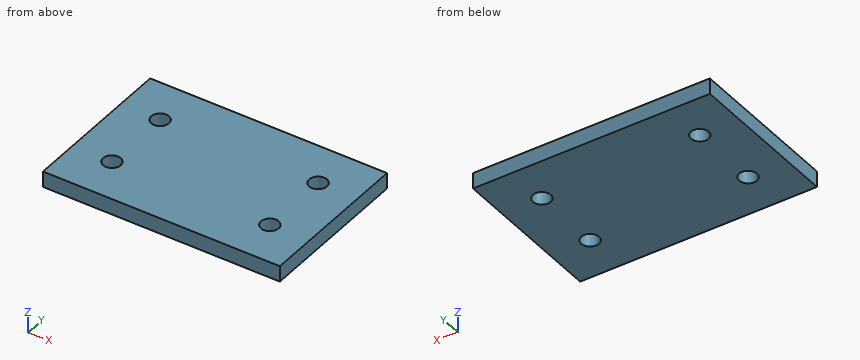
```python
from build123d import *

# Parameters (mm, degrees)
SKETCH_1_W          = 60
SKETCH_1_H          = 40
EXTRUDE_1_DEPTH     = 4
SKETCH_2_R          = 2.25
CUT_EXTRUDE_1_DEPTH = 73.221880341


with BuildPart() as part:
    # 草图1 → 凸台-拉伸1 (new body)
    with BuildSketch(Plane.XY):
        with Locations((30, 20)):
            Rectangle(SKETCH_1_W, SKETCH_1_H)
    extrude(amount=EXTRUDE_1_DEPTH)

    # 草图2 → 切除-拉伸1 (cut, through all)
    with BuildSketch(Plane.XY.offset(4)):
        with Locations((10, 11)):
            Circle(SKETCH_2_R)
        with Locations(Location((50, 11, 0), (0, 0, 180))):
            Circle(SKETCH_2_R)
        with Locations((50, 29)):
            Circle(SKETCH_2_R)
        with Locations(Location((10, 29, 0), (0, 0, 180))):
            Circle(SKETCH_2_R)
    extrude(amount=-CUT_EXTRUDE_1_DEPTH, mode=Mode.SUBTRACT)


solid = part.part
```
Model file for the job. Use its own axes, mm. Round coordinates to 2 decimals unless told otherwise and drop trailing zeros. Write each loop counter-clockwise with the first axis right and the second up, starting at its lowest first coordinate (ties: lowest second). Pieces come first, ordered by that corner, then holes. Notation, with made-up numbers: (36.5, 54) - (51.5, 54) arc R18 cw to (51.5, 73) - close; hole circle Ø5 at (75.5, -36.5). An arc over 180 degrees is marked (long way). One line per item, written item: value.
(1) Drop a flat-ended pin along its axis: P1, Ø1, axis at x = 9.5, y = 9.5, coming from the +Z side. Give the stop position or say it passes through.
Values follow:
P1: passes through
(2) Cut at A-A, the plane z = 2.55. Give the cut face in (x, y).
Values follow:
outline: (0, 0) - (60, 0) - (60, 40) - (0, 40) - close; hole circle Ø4.5 at (10, 11); hole circle Ø4.5 at (10, 29); hole circle Ø4.5 at (50, 11); hole circle Ø4.5 at (50, 29)
(3) Cut at B-B, the plane y = 29. Give the cut face in (x, z), plus the area to 3 significant figures.
Values follow:
outline: (0, 0) - (7.75, 0) - (7.75, 4) - (0, 4) - close; (12.25, 0) - (47.75, 0) - (47.75, 4) - (12.25, 4) - close; (52.25, 0) - (60, 0) - (60, 4) - (52.25, 4) - close
area: 204 mm²
(4) Cut at C-C, the plane x = 10. Give the cut face in (y, z), plus the area to 3 significant figures.
Values follow:
outline: (0, 0) - (8.75, 0) - (8.75, 4) - (0, 4) - close; (13.25, 0) - (26.75, 0) - (26.75, 4) - (13.25, 4) - close; (31.25, 0) - (40, 0) - (40, 4) - (31.25, 4) - close
area: 124 mm²
(5) Wall check: probe 1 along Y at (x, z) = (50, 2.65); probe 2 along X at (y, z) = (27, 0.4). Give the ranges that are in metal, low to high.
Values follow:
probe 1: y = 0 to 8.75, 13.25 to 26.75, 31.25 to 40
probe 2: x = 0 to 8.97, 11.03 to 48.97, 51.03 to 60
